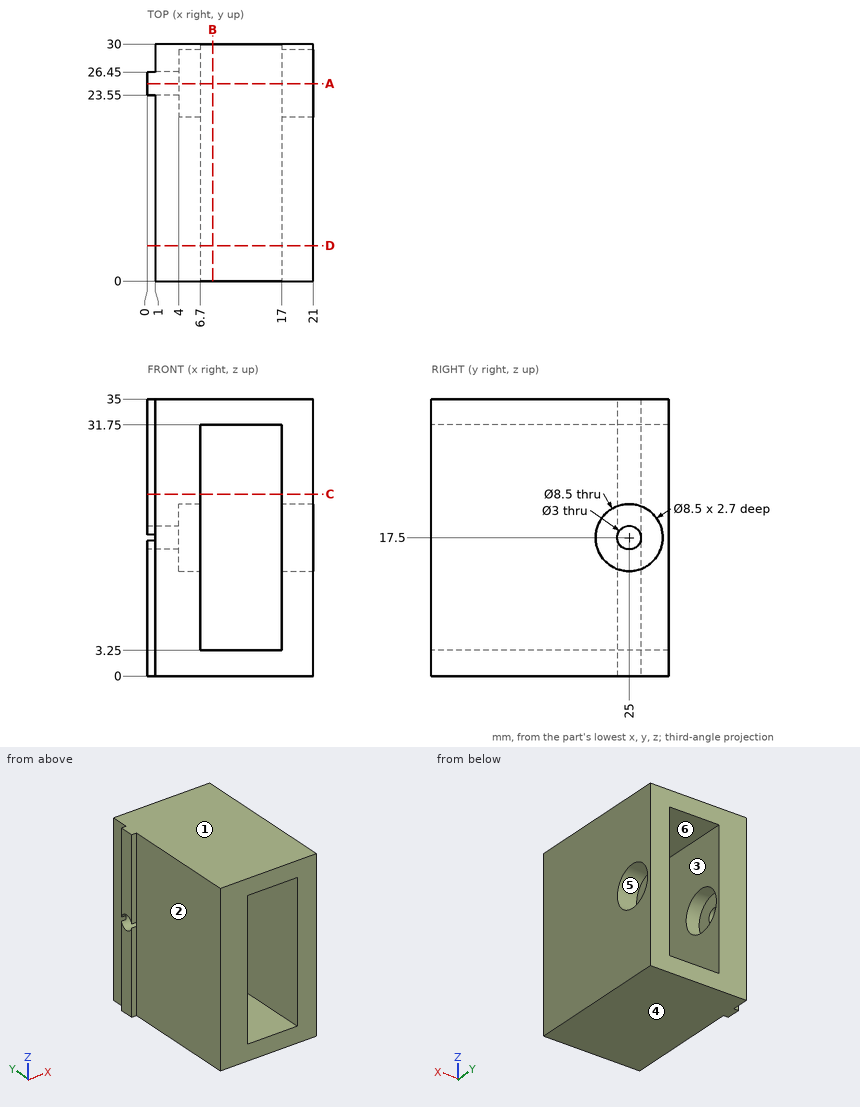
Study the drawing (mm; zero at the part's minimum x, y, z) and answer. A direction names the side the tool comes from. Round coordinates to 2 decimals unless told otherwise and drop trailing zeros. Order: outer loops, then holes, each group sorted by start corner. A loop starts at its lowest first (then second) coordinate and runs counter-clockwise, first axis right, second up. Notation, with made-up numbers: (27.5, -29.75) -> (51.5, -29.75) arc R24 ccw to (51.5, -9.75) -> close; hole circle Ø8 at (-21.75, -1). An arc over 180 degrees is marked (long way). Write each question's results on one line, items separated by ' | '. Start each with the question number.
Q1. Which of the six approach directions +Z, -Z, +X, -X, +Y, -Y give full straight-line access (tool end or side, diameter ignored) to the marked faces 4, 5 and 6?
Q2. Find section B-B (x = 8.25). Determine the outline of the cut face in (y, z).
Q3. Find section A-A (y = 25). Determine the outline of the cut face in (x, z), then the cut area to 4 significant figures.
Q4. Find section D-D (y = 4.5). Determine the outline of the cut face in (x, z).
Q5. Find section C-C (z = 23). Determine the outline of the cut face in (x, y), then the cut area to 3 significant figures.
Q6. Each of these flat-tipped pins is pushed along its axis until it touches: pin 1 (0.8 mm diameter, centred on x = 0.5, z = 7.5, fed in from -Y); pin 2 (1.1 mm diameter, centred on y = 29, z = 10, fed in from -X); pin 3 (2.5 mm diameter, centred on y = 25, z = 17.5, fed in from +X). Where does it stop, or does it pass through?
Q7. Straight lines are drawn through the part: probe 1 along X at (y, z) = (7, 5.5); probe 2 along Z at (x, y) = (9, 12.25); probe 3 along Z at (x, y) = (5.85, 25). For each, find the intervals that lie inside material, in ascending order. Write a range as from..to.
Q8. The mould has two halves that part along Z. Classify the marked faces 1, 2 and 3: pulls with the +Z half, pulls with the -Z half, needs draft (parallel to the pull), parting line crosses it, or undercut.
Worked answers:
1) face 4: -Z, +X, -X, +Y, -Y | face 5: +X | face 6: +Y, -Y
2) outline: (0, 0) -> (30, 0) -> (30, 3.25) -> (0, 3.25) -> close; (0, 31.75) -> (30, 31.75) -> (30, 35) -> (0, 35) -> close
3) outline: (0, 0) -> (21, 0) -> (21, 13.25) -> (17, 13.25) -> (17, 3.25) -> (6.7, 3.25) -> (6.7, 13.25) -> (4, 13.25) -> (4, 16) -> (0, 16) -> close; (0, 19) -> (4, 19) -> (4, 21.75) -> (6.7, 21.75) -> (6.7, 31.75) -> (17, 31.75) -> (17, 21.75) -> (21, 21.75) -> (21, 35) -> (0, 35) -> close | area: 372.5 mm2
4) outline: (1, 0) -> (21, 0) -> (21, 35) -> (1, 35) -> close; hole (6.7, 3.25) -> (17, 3.25) -> (17, 31.75) -> (6.7, 31.75) -> close
5) outline: (0, 23.55) -> (1, 23.55) -> (1, 0) -> (6.7, 0) -> (6.7, 30) -> (1, 30) -> (1, 26.45) -> (0, 26.45) -> close; (17, 0) -> (21, 0) -> (21, 30) -> (17, 30) -> close | area: 294 mm2
6) pin 1: stops at y = 23.55 | pin 2: stops at x = 1 | pin 3: passes through
7) probe 1: x = 1..6.7, 17..21 | probe 2: z = 0..3.25, 31.75..35 | probe 3: z = 0..13.25, 21.75..35
8) face 1: pulls with the +Z half | face 2: needs draft | face 3: undercut
